Part model, mm, in its own coordinate system. Face numbers are marked on the shaded views. A direction names the side the tool comes from. Round coordinates to 2 decimals unless told otherwise and drop trailing zeros. Loops run counter-clockwise (first coordinate to the right, second up) from the corner with the lowest first, then second, coordinate; pieces in that order, holes last.
(1) Flat gauge pins, fed straight in: pin 1 (11.5 mm diameter, centred on x = 76.2, y = 25.4, fed in from +Z); pin 2 (1.5 mm diameter, centred on y = 39, z = 3, fed in from -X); pin 3 (2 mm diameter, centred on y = -5, z = 5, fed in from +X); pin 4 (2 mm diameter, centred on x = 9.5, y = 19, fed in from -Z). Where does each tip first touch, or does it go through?
(2) Probe probe 1 along Y at (x, z) = (20, 1.5); probe 2 along Z at (x, y) = (96.5, 27.5); probe 3 along X at (y, z) = (55, 3.5). List the from-to ranges inside material, lowest first.
(3) Tool access for the marked faces 1 and 2: list every direction of +Z, -Z, +X, -X, +Y, -Y with a clear straight run to the whole face (end or side of a thin tool).
(4) Cut at C-C on y = 66.5. List the corners of the cut face in (x, z), then the cut area to 3 significant figures.
(5) Cut at D-D on x = 119. List the corners of the cut face in (y, z).
(6) Cut at A-A on y = 18. List the corners of the cut face in (x, z).
from build123d import *

# Parameters (mm, degrees)
F1_DEPTH      = 6.35
F2_R          = 2.921
F3_DEPTH      = 102.108
F3_DEPTH_BACK = 25.4
F6_D          = 19.05
F7_W          = 25.4
F7_H          = 8.6004827172
F7_H_2        = 11.8143679574
F8_DEPTH      = 12.7


# Not quite as in the source:
# - a feature names something its author has since deleted; it is built from what else it names


with BuildPart() as f1:
    # F0 (on Top) → F1 (new body)
    with BuildSketch(Plane.XY):
        Polygon((139.7, 95.25), (-63.5, 95.25), (-25.4, 0), (101.6, 0), align=None)
    extrude(amount=F1_DEPTH)

    # F2 (on Right) → F3 (join, two sides)
    with BuildSketch(Plane.YZ) as f3_sk:
        with BuildLine():
            Line((0, 0), (0, 6.337816827))
            ThreePointArc((0, 6.337816827), (-7.4383769178, 3.1689084135), (0, 0))
        make_face()
        with Locations((-3.0441769178, 3.1689084135)):
            Circle(F2_R, mode=Mode.SUBTRACT)
    extrude(amount=F3_DEPTH)
    extrude(f3_sk.sketch, amount=-F3_DEPTH_BACK)

    # F6 (through all)
    with Locations(Plane(origin=(0, 0, 0), x_dir=(1, 0, 0), z_dir=(0, 0, -1))):
        with Locations((0, -25.400012026), (76.2, -25.400012026)):
            Hole(F6_D / 2)

    # F7 (on face) → F8 (cut, symmetric)
    with BuildSketch(Plane.XY.offset(6.35)):
        with Locations((12.7, -4.3002413586)):
            Rectangle(F7_W, F7_H)
        with Locations((63.5, -5.9071839787)):
            Rectangle(F7_W, F7_H_2)
    extrude(amount=F8_DEPTH, both=True, mode=Mode.SUBTRACT)


solid = f1.part
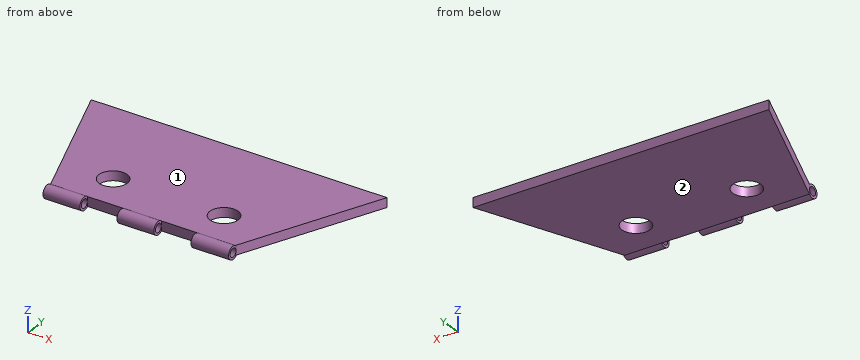
Final values:
1. pin 1: passes through
1. pin 2: stops at x = -41.3
1. pin 3: stops at x = 102.11
1. pin 4: stops at z = 0
2. probe 1: y = 0 to 95.25
2. probe 2: z = 0 to 6.35
2. probe 3: x = -47.4 to 123.6
3. face 1: +Z, +X, -X, +Y
3. face 2: -Z, +X, -X, +Y
4. outline: (-52, 0) - (128.2, 0) - (128.2, 6.35) - (-52, 6.35) - close
4. area: 1,140 mm2
5. outline: (43.5, 0) - (95.25, 0) - (95.25, 6.35) - (43.5, 6.35) - close
6. outline: (-32.6, 0) - (-6, 0) - (-6, 6.35) - (-32.6, 6.35) - close; (6, 0) - (70.2, 0) - (70.2, 6.35) - (6, 6.35) - close; (82.2, 0) - (108.8, 0) - (108.8, 6.35) - (82.2, 6.35) - close
